Build history of the part. All positions in model axes, mm. A direction names the side the tool comes from. Coordinates: 2 decimals unless noted, no trailing zeros. Order: outer loops, then holes, each group sorted by start corner. A loop starts at its lowest first (then second) coordinate and runs counter-clockwise, first axis right, second up. Notation, with made-up numbers: (29.25, -12) - (79.25, -12) arc R29 cw to (79.25, 19) - close; hole circle Ø9 at (-10, 83). An arc over 180 degrees is marked (long way). Return JSON: item names as keys, results as strings.
from build123d import *

# Parameters (mm, degrees)
BASE_DEPTH      = 50.8
AXLE_HOLE_REACH = 23.59
SKETCH2_R       = 4


with BuildPart() as part:
    # Sketch1 → base (new body)
    with BuildSketch(Plane.XY):
        Polygon((-26.940768363, 26.940768363), (0, 0), (25.4, 0), (25.4, 2.54), (1.052102448, 2.54), (-25.144717139, 28.736819587), align=None)
    extrude(amount=BASE_DEPTH)

    # Sketch2 → axle hole (cut, up to next)
    with BuildSketch(Plane(origin=(1.796051224, 1.796051224, 0), x_dir=(0, 0, -1), z_dir=(0.707106781, 0.707106781, 0)), mode=Mode.PRIVATE) as axle_hole_sk1:
        with Locations((-19.05, 19.576051224)):
            Circle(SKETCH2_R)
    axle_hole_tool1 = extrude(axle_hole_sk1.sketch, amount=-AXLE_HOLE_REACH, mode=Mode.PRIVATE) & part.part
    add(axle_hole_tool1.solids().sort_by_distance((-12.046307, 15.63841, 19.05))[0], mode=Mode.SUBTRACT)


solid = part.part
1. Mould opens along Z. For faces 3 (the cylindrical face through (-13.056, 14.877, 23.046)), 4 (the flat face through (25.4, 1, 25)), 5 (the flat face through (-5, 8, 0)) say: pulls with the +Z half, pulls with the -Z half, needs draft (parallel to the pull), parting line crosses it, or undercut.
Check values:
{"face 3": "undercut", "face 4": "needs draft", "face 5": "pulls with the -Z half"}
2. Drop flat-ended pins along their axis: pin 1 (1.5 mm diameter, centred on x = -4.5, z = 14.5, fed in from -Y); pin 2 (2 mm diameter, centred on y = 23.5, z = 40.5, fed in from +X); pin 3 (4 mm diameter, centred on x = -3, y = 10.5, fed in from +Z); pin 4 (1.5 mm diameter, centred on y = 6, z = 7.5, fed in from -X). Give the stop position or say it passes through.
Check values:
{"pin 1": "y = 3.75", "pin 2": "x = -18.91", "pin 3": "through", "pin 4": "x = -6.75"}
3. Tool access for faces 1 (the flat face through (-5, 8, 50.8)), 2 (the flat face through (13, 2.54, 25)): list every direction of +Z, -Z, +X, -X, +Y, -Y with a clear straight run to the whole face (end or side of a thin tool).
Check values:
{"face 1": "+Z, +X, -X, +Y, -Y", "face 2": "+Z, -Z, +X, +Y"}
4. Cut at C-C on y = 7. Give the cut face in (x, z).
Check values:
{"outline": "(-7, 0) - (-3.41, 0) - (-3.41, 50.8) - (-7, 50.8) - close"}
5. Cut at B-B on x = 9. Give the cut face in (y, z), plus the area to 3 significant figures.
Check values:
{"outline": "(0, 0) - (2.54, 0) - (2.54, 50.8) - (0, 50.8) - close", "area": "129 mm²"}
6. Probe L1, parallel to Y at x = 17.5, z = 46; L2, parallel to X at y = 3, z = 27; L3, parallel to X at y = 19.25, z = 25. List the from-to ranges inside material, lowest first.
Check values:
{"L1": "0 to 2.54", "L2": "-3 to 0.59", "L3": "-19.25 to -15.66"}
7. Cut at A-A on z = 41. Give the cut face in (x, y), plus the area to 3 significant figures.
Check values:
{"outline": "(-26.94, 26.94) - (0, 0) - (25.4, 0) - (25.4, 2.54) - (1.05, 2.54) - (-25.14, 28.74) - close", "area": "159 mm²"}
